For this review, take the finished solid that the model builds, in its own axes (mm). Give positions to 0.01 mm unless a question says otherwise; leave off trailing zeros. Write each loop counter-clockwise with the first axis right and the second up, starting at its lowest first coordinate (ties: lowest second). Pieces come first, ordered by that corner, then holes. Notation, with made-up numbers: M 66.5,19 L 92.5,19 A36 ccw 92.5,57 Z; hole C -29,68 d9. An arc over 180 degrees is marked long. Write item = value, one per line.
```python
from build123d import *

# Parameters (mm, degrees)
BOSS_EXTRU_1_DEPTH      = 2
ESQUISSE2_RX            = 10
ESQUISSE2_RY            = 6.5
ENL_V_MAT_EXTRU_1_DEPTH = 69.410525506
ESQUISSE3_R             = 1.55
ESQUISSE3_R_2           = 1.6
ESQUISSE3_R_3           = 1.25
ENL_V_MAT_EXTRU_2_DEPTH = 10


with BuildPart() as part:
    # Esquisse1 → Boss.-Extru.1 (new body)
    with BuildSketch(Plane(origin=(0, 0, 0), x_dir=(1, 0, 0), z_dir=(0, 1, 0))):
        with BuildLine():
            Line((-46.647615159, 18), (-40, 18))
            ThreePointArc((-40, 18), (-38.585786438, 17.414213562), (-38, 16))
            Line((-38, 16), (-38, -16))
            ThreePointArc((-38, -16), (-38.585786438, -17.414213562), (-40, -18))
            Line((-40, -18), (-46.647615159, -18))
            ThreePointArc((-46.647615159, -18), (0, -50), (46.647615159, -18))
            Line((46.647615159, -18), (40, -18))
            ThreePointArc((40, -18), (38.585786438, -17.414213562), (38, -16))
            Line((38, -16), (38, 16))
            ThreePointArc((38, 16), (38.585786438, 17.414213562), (40, 18))
            Line((40, 18), (46.647615159, 18))
            ThreePointArc((46.647615159, 18), (0, 50), (-46.647615159, 18))
        make_face()
    extrude(amount=BOSS_EXTRU_1_DEPTH)

    # Esquisse2 → Enlèv. mat.-Extru.1 (cut, through all)
    with BuildSketch(Plane(origin=(0, 2, 0), x_dir=(1, 0, 0), z_dir=(0, 1, 0))):
        with Locations((0, 40)):
            Ellipse(ESQUISSE2_RX, ESQUISSE2_RY)
        with Locations((0, -40)):
            Ellipse(ESQUISSE2_RX, ESQUISSE2_RY)
    extrude(amount=-ENL_V_MAT_EXTRU_1_DEPTH, mode=Mode.SUBTRACT)

    # Esquisse3 → Enlèv. mat.-Extru.2 (cut)
    with BuildSketch(Plane(origin=(0, 2, 0), x_dir=(1, 0, 0), z_dir=(0, 1, 0))):
        with Locations(Location((-30, 30, 0), (0, 0, 270))):
            Circle(ESQUISSE3_R)
        with Locations(Location((30, 30, 0), (0, 0, 90))):
            Circle(ESQUISSE3_R)
        with Locations(Location((30, -30, 0), (0, 0, 270))):
            Circle(ESQUISSE3_R)
        with Locations(Location((-30, -30, 0), (0, 0, 90))):
            Circle(ESQUISSE3_R)
        with Locations(Location((-15, 40, 0), (0, 0, 270))):
            Circle(ESQUISSE3_R_2)
        with Locations(Location((15, 40, 0), (0, 0, 90))):
            Circle(ESQUISSE3_R_2)
        with Locations(Location((15, -40, 0), (0, 0, 270))):
            Circle(ESQUISSE3_R_2)
        with Locations(Location((-15, -40, 0), (0, 0, 90))):
            Circle(ESQUISSE3_R_2)
        with Locations(Location((-34, 9, 0), (0, 0, 270))):
            Circle(ESQUISSE3_R_3)
        with Locations(Location((-34, -9, 0), (0, 0, 90))):
            Circle(ESQUISSE3_R_3)
        with Locations(Location((34, -9, 0), (0, 0, 270))):
            Circle(ESQUISSE3_R_3)
        with Locations(Location((34, 9, 0), (0, 0, 90))):
            Circle(ESQUISSE3_R_3)
    extrude(amount=-ENL_V_MAT_EXTRU_2_DEPTH, mode=Mode.SUBTRACT)


solid = part.part
```
1. We need section D-D, the plane z = -22. Write out the cut boundary in (x, y), then the cut area to 3 significant figures.
Responses:
outline = M -44.9,0 L 44.9,0 L 44.9,2 L -44.9,2 Z
area = 180 mm2
2. We need section C-C, the plane z = -5. Write out the cut boundary in (x, y).
Responses:
outline = M -38,0 L 38,0 L 38,2 L -38,2 Z
3. Insertion check: P1, Ø0.6, axis at y = 1, z = -4.5, coming from the +X side; P2, Ø1, axis at x = 42.5, y = 1, coming from the -Z side; P3, Ø1, axis at x = -44.5, y = 1.5, coming from the -Z side. Each pin has a flat end and moves straight along its axis. Give the tip position at first contact, or say it passes through.
Responses:
P1 = 38
P2 = -27.13
P3 = -23.75
4. The part is to be moulded in two halves that separate along Z. For faces 1 (the face through (33.95, 1.01, -7.75)), 2 (the face through (0.842, 0.986, -49.993)), 3 (the face through (-1, 0, -1)), say which applies: +Z half, -Z half, draft (parallel to the pull), parting line (faces both ways), or undercut.
Responses:
face_1 = undercut
face_2 = -Z half
face_3 = draft
5. For line 1 along X through (y, z) = (1.3, -9); line 2 along X through (y, z) = (1.2, 30); line 3 along Z through (x, y) = (31, 1.85), list the stretches that pass through material, from the lowest coordinate up. Write a range as from..to.
Responses:
line_1 = -38..-35.25, -32.75..32.75, 35.25..38
line_2 = -40..-31.55, -28.45..28.45, 31.55..40
line_3 = -39.23..-31.18, -28.82..28.82, 31.18..39.23
6. We need section B-B, the plane x = -30. Write out the cut boundary in (y, z).
Responses:
outline = M 0,-40 L 2,-40 L 2,-31.55 L 0,-31.55 Z; M 0,-28.45 L 2,-28.45 L 2,28.45 L 0,28.45 Z; M 0,31.55 L 2,31.55 L 2,40 L 0,40 Z
7. We need section A-A, the plane z = 30. Write out the cut boundary in (x, y).
Responses:
outline = M -40,0 L -31.55,0 L -31.55,2 L -40,2 Z; M -28.45,0 L 28.45,0 L 28.45,2 L -28.45,2 Z; M 31.55,0 L 40,0 L 40,2 L 31.55,2 Z
